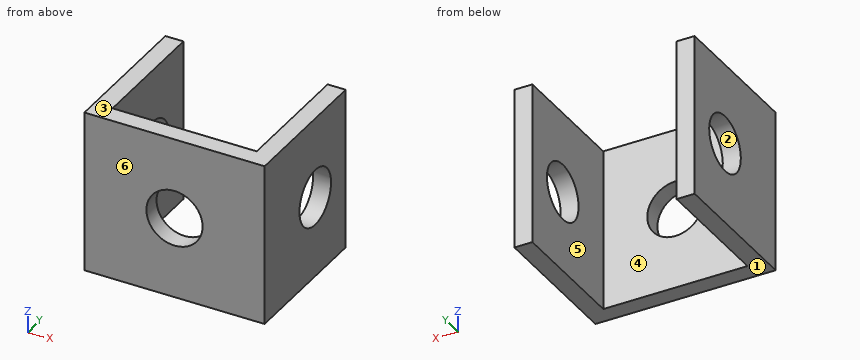
from build123d import *

# Parameters (mm, degrees)
SKETCH1_W           = 50
SKETCH1_H           = 45
BOSS_EXTRUDE1_DEPTH = 5
SKETCH5_W           = 5
SKETCH5_H           = 45
BOSS_EXTRUDE3_DEPTH = 35
SKETCH9_R           = 7.8
CUT_EXTRUDE5_DEPTH  = 10
SKETCH11_R          = 7.8
CUT_EXTRUDE8_DEPTH  = 51


with BuildPart() as part:
    # Sketch1 → Boss-Extrude1 (new body)
    with BuildSketch(Plane(origin=(0, 0, 0), x_dir=(1, 0, 0), z_dir=(0, 1, 0))):
        Rectangle(SKETCH1_W, SKETCH1_H)
    extrude(amount=BOSS_EXTRUDE1_DEPTH)

    # Sketch5 → Boss-Extrude3 (add)
    with BuildSketch(Plane(origin=(0, 5, 0), x_dir=(1, 0, 0), z_dir=(0, 1, 0))):
        with Locations((22.5, 0)):
            Rectangle(SKETCH5_W, SKETCH5_H)
        with Locations((-22.5, 0)):
            Rectangle(SKETCH5_W, SKETCH5_H)
    extrude(amount=BOSS_EXTRUDE3_DEPTH)

    # Sketch9 → Cut-Extrude5 (cut)
    with BuildSketch(Plane(origin=(0, 5, 0), x_dir=(1, 0, 0), z_dir=(0, 1, 0))):
        Circle(SKETCH9_R)
    extrude(amount=-CUT_EXTRUDE5_DEPTH, mode=Mode.SUBTRACT)

    # Sketch11 → Cut-Extrude8 (cut, through all)
    with BuildSketch(Plane.ZY.offset(25)):
        with Locations((0, 25)):
            Circle(SKETCH11_R)
    extrude(amount=-CUT_EXTRUDE8_DEPTH, mode=Mode.SUBTRACT)


solid = part.part
Here's how the part is built. I have some questions about the finished solid (model axes, mm). Face numbers are marked on the shaded views. A direction names the side the tool comes from. Round coordinates to 2 decimals unless told otherwise and drop trailing zeros. Write each loop counter-clockwise with the first axis right and the second up, starting at its lowest first coordinate (ties: lowest second). Pieces come first, ordered by that corner, then holes.
1. Suppose I cut it at C-C (z = 0). List the corners of the cut face in (x, y) for me.
2. I need wall thicknesses on L1, parallel to X at y = 3, z = 0; L2, parallel to X at y = 36, z = -11.5; L3, parallel to Y at x = 21.4, z = 0. Which ranges of each line are inside material? Lowest first, please.
3. Suppose I cut it at B-B (y = 25). List the corners of the cut face in (x, z) for me, and give its area (3 significant figures).
4. For the marked faces 5 and 6, which set-ups out of +Z, -Z, +X, -X, +Y, -Y let a thin tool reach every point of the face, with its end or its side?
5. Will this pin go through, and if not, where does the flat tip stop? pin 1 Ø9.5 at (x, z) = (0, 0) entering from +Y.
6. Suppose I cut it at D-D (x = 21). List the corners of the cut face in (y, z) for me.
7. Suppose I cut it at A-A (x = 0). List the corners of the cut face in (y, z) for me.
8. If we mould it in two halves opening along Z, with no side actions, what happens to the marked faces 1, 2, 3 and 4? For each: released by +Z, released by -Z, zero draft, split by the parting line, or undercut.
Answer sheet:
1. outline: (-25, 0) - (-7.8, 0) - (-7.8, 5) - (-20, 5) - (-20, 17.2) - (-25, 17.2) - close; (-25, 32.8) - (-20, 32.8) - (-20, 40) - (-25, 40) - close; (7.8, 0) - (25, 0) - (25, 17.2) - (20, 17.2) - (20, 5) - (7.8, 5) - close; (20, 32.8) - (25, 32.8) - (25, 40) - (20, 40) - close
2. L1: x = -25 to -7.8, 7.8 to 25
2. L2: x = -25 to -20, 20 to 25
2. L3: y = 0 to 17.2, 32.8 to 40
3. outline: (-25, -22.5) - (-20, -22.5) - (-20, -7.8) - (-25, -7.8) - close; (-25, 7.8) - (-20, 7.8) - (-20, 22.5) - (-25, 22.5) - close; (20, -22.5) - (25, -22.5) - (25, -7.8) - (20, -7.8) - close; (20, 7.8) - (25, 7.8) - (25, 22.5) - (20, 22.5) - close
3. area: 294 mm2
4. face 5: +Z, -Z, +Y
4. face 6: +Z, -Z, +X, -X, -Y
5. pin 1: passes through
6. outline: (0, -22.5) - (40, -22.5) - (40, 22.5) - (0, 22.5) - close; hole circle Ø15.6 at (25, 0)
7. outline: (0, -22.5) - (5, -22.5) - (5, -7.8) - (0, -7.8) - close; (0, 7.8) - (5, 7.8) - (5, 22.5) - (0, 22.5) - close
8. face 1: released by -Z
8. face 2: undercut
8. face 3: released by +Z
8. face 4: zero draft
